For this review, use the dimensioned drawing (mm, ordinates from the lowest corner) and the shaded views. A direction names the side the tool comes from. Coordinates: 2 decimals unless noted, no trailing zeros. Loops run counter-clockwise (first coordinate to the right, second up) from the corner with the lowest first, then second, coordinate; pieces in that order, holes last.
1. Take a section at B-B, the plane y = 6.75. State the section outline as (x, z) points.
2. Mouldability with a two-part tool opening along X and no side actions: class the marked faces 3, 4, 5 and 6 as pulls with the +X half, pulls with the -X half, needs draft (parallel to the pull), parting line crosses it, or undercut.
3. To check wall thickness, follow probe 1 along X at (y, z) = (7.75, 17); probe 2 along X at (y, z) = (0.35, 5); probe 3 along Z at (x, y) = (4.5, 2.25) (1 decimal). State the ranges of each line that lie inside material, in increasing order.
4. Machinability: for the marked faces 1 and 2, which of the approach directions +Z, -Z, +X, -X, +Y, -Y give a long, thin tool a straight path to every point of the face, cutting with its end or side? Answer none if there is none.
5. Take a section at D-D, the plane x = 7.94. State the section outline as (y, z) points.
6. Clearance check with flat-ended pins moving along their axes: P1, Ø7, axis at x = 7.94, z = 5, coming from the -Y side; P2, Ø4, axis at x = 11, z = 38.5, coming from the +Y side; P3, Ø3.5, axis at x = 10, y = 15, coming from the +Z side; P4, Ø3.5, axis at x = 7.94, z = 17, coming from the +Y side. State where each tip first meets the part, or that it passes through.
7. Take a section at C-C, the plane x = 1. State the section outline as (y, z) points.
8. Take a section at A-A, the plane z = 17. State the section outline as (x, y) points.
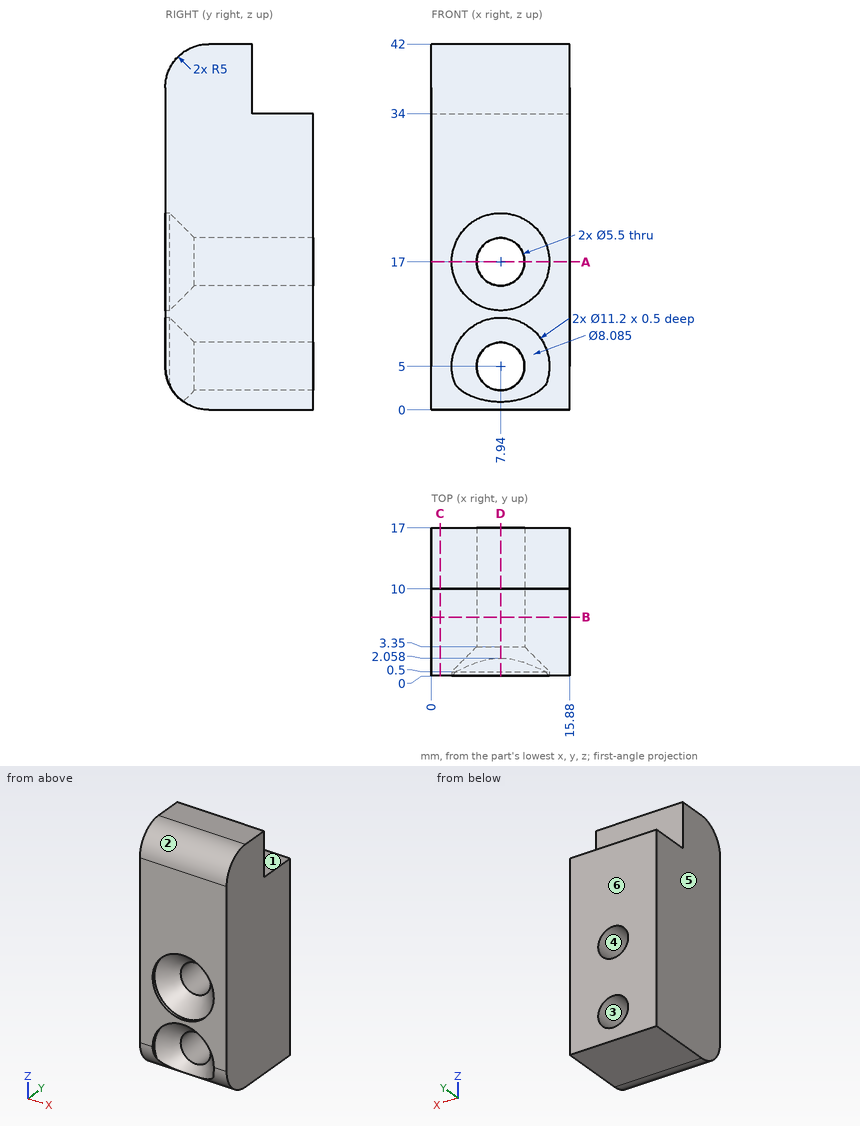
Results list:
1. outline: (0, 0) - (15.88, 0) - (15.88, 42) - (0, 42) - close; hole circle Ø5.5 at (7.94, 5); hole circle Ø5.5 at (7.94, 17)
2. face 3: undercut
2. face 4: undercut
2. face 5: pulls with the -X half
2. face 6: needs draft
3. probe 1: x = 0 to 5.19, 10.69 to 15.88
3. probe 2: x = 0 to 2.34, 13.54 to 15.88
3. probe 3: z = 0.8 to 3.3, 6.7 to 15.3, 18.7 to 41.2
4. face 1: +Z, +X, -X, +Y
4. face 2: +Z, +X, -X, -Y
5. outline: (0, 10.6) - (0.5, 10.6) - (3.35, 7.75) - (17, 7.75) - (17, 14.25) - (3.35, 14.25) - (0.5, 11.4) - (0, 11.4) - close; (0, 22.6) - (0.5, 22.6) - (3.35, 19.75) - (17, 19.75) - (17, 34) - (10, 34) - (10, 42) - (5, 42) arc R5 ccw to (0, 37) - close; (2.06, 0.96) arc R5 ccw to (5, 0) - (17, 0) - (17, 2.25) - (3.35, 2.25) - close
6. P1: stops at y = 2.6
6. P2: stops at y = 10
6. P3: stops at z = 34
6. P4: passes through
7. outline: (0, 5) arc R5 ccw to (5, 0) - (17, 0) - (17, 34) - (10, 34) - (10, 42) - (5, 42) arc R5 ccw to (0, 37) - close
8. outline: (0, 0) - (2.34, 0) - (2.34, 0.5) - (5.19, 3.35) - (5.19, 17) - (0, 17) - close; (10.69, 3.35) - (13.54, 0.5) - (13.54, 0) - (15.88, 0) - (15.88, 17) - (10.69, 17) - close
